Can you work these out from the model? Positions are in its coordinate system, mm. A direction names the side the tool comes from. Round coordinates to 2 decimals unless told otherwise and drop trailing zeros. Write each loop counter-clockwise with the first axis right and the second up, starting at its lowest first coordinate (ties: lowest second). Pieces come first, ordered by that corner, then holes. Notation, with made-up numbers: (74.25, -15.75) -> (113.25, -15.75) arc R22 ccw to (113.25, 22.25) -> close; hole circle Ø1 at (-7, 37.25). An arc over 180 degrees is marked (long way). Write item = value, one per line. Start each with the question number.
1) Imagine slicing it at A-A, the plane x = 1. Please give me the cut outline in (y, z), then the cut area to 3 significant figures.
2) Thinking about a two-plate mould opening in Y: for faces 1 (the face through (10, 0, 0)), 2 (the face through (1.992, -1.345, -0.059)), 3 (the face through (0.867, -1.168, -0.003)), which applies, +Y half, -Y half, draft (parallel to the pull), parting line (faces both ways), or undercut?
3) I'm going to push flat-ended pins straight in: pin 1 (1 mm diameter, centred on x = 2.5, y = 0.5, fed in from -Z); pin 2 (1 mm diameter, centred on y = -1, z = -1.5, fed in from +X); pin 3 (1.5 mm diameter, centred on x = 6.5, z = 2, fed in from -Y). Where does each tip first touch, or does it pass through?
4) For faces 4 (the face through (0, 1, -1)), 5 (the face through (0.867, 1.168, 0.003)), which set-ups out of +Z, -Z, +X, -X, +Y, -Y let a thin tool reach every point of the face, with its end or its side?
5) If I drill on line 1 (X direction, y = -1.4, z = -0.4); line 2 (Y direction, x = 0.75, z = -0.55); line 3 (Y direction, x = 8.5, z = 0.1), over which ranges is the centre line in solid material (lowest first)?
6) Imagine slicing it at B-B, the plane x = 9. Please give me the cut outline in (y, z), then the cut area to 3 significant figures.
Autodesk Inventor part; units mm, degrees
ref_plane "Work Plane2" through (3.35, 0, 0) normal (0, 0, -1) x (1, 0, 0)
ref_plane "YZ Plane" through (0, 0, 0) normal (1, 0, 0) x (0, 1, 0)
ref_plane "XZ Plane" through (0, 0, 0) normal (0, 1, 0) x (-1, 0, 0)
sketch "Szkic1" plane through (0, 0, 0) normal (0, 0, 1) x (1, 0, 0)
  line L0 (2.1, 0) -> (10, 0)
  line L1 (10, 0) -> (10, 1.5)
  line L2 (10, 1.5) -> (2.65, 1.5)
  line L3 (2.65, 1.5) -> (2.3433, 1.3466)
  line L4 (2.3433, 1.3466) -> (1.65, 1.3466)
  line L5 (0, 2.75) -> (0, 1.6)
  line L6 (0, 1.6) -> (1.6999, 0.7525)
  line L7 (1.6999, 0.7525) -> (2.1, 0)
  line L8 (-2, 0) -> (12, 0)
  line L9 (0, -0.55) -> (0, 3.3)
  line L10 (0, 2.75) -> (0.2466, 2.75)
  line L11 (0.2466, 2.75) -> (1.65, 1.3466)
  line L12 (2.65, 1.5) -> (1.4966, 1.5) construction
  dimension "d1" = 7.35
  dimension "d2" = 3
  dimension "d3" = 2.6933
  dimension "d4" = 3.2
  dimension "d5" = 26.5
  dimension "d6" = 62
  dimension "d7" = 2.1
  dimension "d8" = 0.3067
  dimension "d12" = 5.5
  dimension "d13" = 45
  dimension "d15" = 10
  dimension "d24" = 1.65
revolve "Bryła" add sketch "Szkic1" angle 360 about axis through (2.1, 0, 0) along (1, 0, 0) contours L7 L6 L5 L10 L11 L4 L3 L2 L1 L0
sketch "Szkic2" plane through (0, 0, 0) normal (-1, 0, 0) x (0, 0, 1)
  line L0 (0, 1.6) -> (0, 0) construction
  line L1 (0, 0) -> (1.6, 0) construction
  arc A0 (0.48, 0) -> (0, 0.48) centre (0, 0) ccw construction
  arc A1 (0.56, 0) -> (0, 0.56) centre (0, 0) ccw construction
  arc A2 (1.5795, 0.255) -> (0.255, 1.5795) centre (0, 0) ccw
  line L2 (0, 0) -> (1.1314, 1.1314) construction
  line L3 (0.255, 1.5795) -> (0.2766, 0.4869)
  line L4 (1.5795, 0.255) -> (0.4869, 0.2766)
  arc A3 (0.255, 1.5795) -> (0, 1.6) centre (0, 0) ccw
  arc A4 (1.6, 0) -> (1.5795, 0.255) centre (0, 0) ccw
  line L5 (0, -3.85) -> (0, 3.85)
  line L6 (-3.85, 0) -> (3.85, 0)
  arc A5 (0.255, -1.5795) -> (1.5795, -0.255) centre (0, 0) ccw
  line L7 (0.255, -1.5795) -> (0.2766, -0.4869)
  line L8 (1.5795, -0.255) -> (0.4869, -0.2766)
  arc A6 (0, -1.6) -> (0.255, -1.5795) centre (0, 0) ccw
  arc A7 (1.5795, -0.255) -> (1.6, 0) centre (0, 0) ccw
  arc A8 (-0.255, 1.5795) -> (-1.5795, 0.255) centre (0, 0) ccw
  line L9 (-0.255, 1.5795) -> (-0.2766, 0.4869)
  line L10 (-1.5795, 0.255) -> (-0.4869, 0.2766)
  arc A9 (0, 1.6) -> (-0.255, 1.5795) centre (0, 0) ccw
  arc A10 (-1.5795, 0.255) -> (-1.6, 0) centre (0, 0) ccw
  arc A11 (-0.255, -1.5795) -> (0, -1.6) centre (0, 0) ccw
  arc A12 (-1.5795, -0.255) -> (-0.255, -1.5795) centre (0, 0) ccw
  arc A13 (-1.6, 0) -> (-1.5795, -0.255) centre (0, 0) ccw
  line L11 (-1.5795, -0.255) -> (-0.4869, -0.2766)
  line L12 (-0.255, -1.5795) -> (-0.2766, -0.4869)
  arc A14 (0.2766, 0.4869) -> (0.4869, 0.2766) centre (0.4912, 0.4912) ccw
  arc A15 (0.4869, -0.2766) -> (0.2766, -0.4869) centre (0.4912, -0.4912) ccw
  arc A16 (-0.4869, 0.2766) -> (-0.2766, 0.4869) centre (-0.4912, 0.4912) ccw
  arc A17 (-0.2766, -0.4869) -> (-0.4869, -0.2766) centre (-0.4912, -0.4912) ccw
  point P0 (1.1314, -1.1314)
  point P1 (-1.1314, 1.1314)
  point P2 (-1.1314, -1.1314)
  dimension "d17" = 0.96
  dimension "d18" = 1.12
  dimension "d19" = 3.2
  dimension "d20" = 45
  dimension "d21" = 0.255
extrude "Szczelina" add sketch "Szkic2" against normal up to next draft 5 contours L4 A14 L3 A2 | A5 L7 A15 L8 | L9 A16 L10 A8 | A12 L11 A17 L12
fillet "Zaokrąglenie1" radius 0.102 4 edges at (0, 1.6, 0) (0, 0, -1.6) (0, -1.6, 0) (0, 0, 1.6)
thread "Gwint"
chamfer "Faza1" distance 0.3067 distance2 0.1534 1 edges at (10, -1.5, 0) measured on face at (10, -0.5112, 0.3316)
ref_plane "Work Plane2" through (3.35, 0, 0) normal (0, 0, -1) x (1, 0, 0)
equation "\"d1\" = GEL"
equation "\"d2\" = GD"
equation "\"d3\" = BDM"
equation "\"d4\" = SDM"
equation "\"d7\" = INTI"
equation "\"d8\" = GAL"
equation "\"d12\" = KOD"
equation "\"d13\" = 0.5 * SEWI"
equation "\"d15\" = NLG"
equation "\"d24\" = KOH"
equation "\"d17\" = 0.3 * SDM"
equation "\"d18\" = 0.35 * SDM"
equation "\"d19\" = SDM"
equation "\"d21\" = 0.5 * SBR"
equation "\"d23\" = 0.2 * SBR"
equation "\"d10\" = GEL"
equation "\"d25\" = -0.5 * SPD + 0.5 * GD"
equation "\"d26\" = 0.5 * GAL"
equation "\"NLG\" = 10"
equation "\"GEL\" = 7.35"
equation "\"GAL\" = 0.61345 * PTC"
equation "\"SPD\" = NND - 1.2269 * PTC"
equation "\"KOD\" = 5.5"
equation "\"KOH\" = 1.65"
equation "\"SBR\" = 0.51"
equation "\"INTI\" = 2.1"
equation "\"SDM\" = 3.2"
equation "\"GD\" = NND"
equation "\"BDM\" = NND - GAL"
equation "\"SEWI\" = 90deg"
equation "\"d9\" = SDM"
equation "\"GUL\" = 0.61345 * PTC"
equation "\"TOA\" = 30deg"
equation "\"EPV\" = 3.15"
equation "\"THREADDIA\" = 3"
equation "\"PTC\" = 0.5"
equation "\"NND\" = 3"
equation "\"GD1\" = THREADDIA - 1.2269 * PTC"
properties part number "ISO 7046-1 - M3 x 10 - 4.8 - H" material "Stal"
Reported:
q1.outline = circle Ø3.99 at (0, 0); hole (-1.09, -0.18) -> (-0.49, -0.19) arc R0.3 cw to (-0.19, -0.49) -> (-0.18, -1.09) arc R1.1 ccw to (0.18, -1.09) -> (0.19, -0.49) arc R0.3 cw to (0.49, -0.19) -> (1.09, -0.18) arc R1.1 ccw to (1.09, 0.18) -> (0.49, 0.19) arc R0.3 cw to (0.19, 0.49) -> (0.18, 1.09) arc R1.1 ccw to (-0.18, 1.09) -> (-0.19, 0.49) arc R0.3 cw to (-0.49, 0.19) -> (-1.09, 0.18) arc R1.1 ccw to start
q1.area = 11.0 mm²
q2.face_1 = draft
q2.face_2 = parting line
q2.face_3 = undercut
q3.pin_1 = -1.5
q3.pin_2 = 9.95
q3.pin_3 = -0.83
q4.face_4 = +Z, -Z, -X, +Y, -Y
q4.face_5 = -X
q5.line_1 = 0 to 1.54, 2.56 to 9.87
q5.line_2 = -2.18 to -0.21, 0.21 to 2.18
q5.line_3 = -1.5 to 1.5
q6.outline = circle Ø3 at (0, 0)
q6.area = 7.07 mm²
